Check sheet for the modelled part. Datum: model origin and axes. Units: mm. A direction names the side the tool comes from. Round coordinates to 2 decimals unless told otherwise and drop trailing zeros. Write each loop counter-clockwise with the first axis right and the second up, starting at its lowest first coordinate (ties: lowest second). Pieces come first, ordered by that corner, then holes.
from build123d import *

# Parameters (mm, degrees)
SKETCH1_W           = 91
SKETCH1_H           = 91
SKETCH1_W_2         = 85
SKETCH1_H_2         = 85
BOSS_EXTRUDE1_DEPTH = 40
SKETCH2_W           = 91
SKETCH2_H           = 91
BOSS_EXTRUDE2_DEPTH = 3
FILLET1_R           = 2
SKETCH3_R           = 2.5
BOSS_EXTRUDE3_DEPTH = 3


with BuildPart() as part:
    # Sketch1 → Boss-Extrude1 (new body)
    with BuildSketch(Plane(origin=(0, 0, 0), x_dir=(1, 0, 0), z_dir=(0, 1, 0))):
        with Locations((-42.5, 42.5)):
            Rectangle(SKETCH1_W, SKETCH1_H)
        with Locations((-42.5, 42.5)):
            Rectangle(SKETCH1_W_2, SKETCH1_H_2, mode=Mode.SUBTRACT)
    extrude(amount=BOSS_EXTRUDE1_DEPTH)

    # Sketch2 → Boss-Extrude2 (add)
    with BuildSketch(Plane(origin=(0, 40, 0), x_dir=(1, 0, 0), z_dir=(0, 1, 0))):
        with Locations((-42.5, 42.5)):
            Rectangle(SKETCH2_W, SKETCH2_H)
    extrude(amount=BOSS_EXTRUDE2_DEPTH)

    # Fillet1
    fillet1_edges = [part.edges().sort_by_distance(p)[0] for p in [
        (3, 21.5, -88),
        (3, 21.5, 3),
        (-88, 21.5, 3),
        (-88, 21.5, -88),
    ]]
    fillet(fillet1_edges, radius=FILLET1_R)

    # Sketch3 → Boss-Extrude3 (add)
    with BuildSketch(Plane.XZ.offset(-40)):
        with Locations(Location((-66.5, -29.5, 0), (0, 0, 270))):
            Circle(SKETCH3_R)
        with Locations(Location((-66.5, -55.5, 0), (0, 0, 90))):
            Circle(SKETCH3_R)
        with Locations(Location((-18.5, -55.5, 0), (0, 0, 270))):
            Circle(SKETCH3_R)
        with Locations(Location((-18.5, -29.5, 0), (0, 0, 90))):
            Circle(SKETCH3_R)
    extrude(amount=BOSS_EXTRUDE3_DEPTH)


solid = part.part
1. Sectioned sample at C-C, the plane z = -72.5. Enter the section's corners in (x, y).
2. Sectioned sample at B-B, the plane x = -66.5. Enter the section's corners in (y, z).
3. Sectioned sample at D-D, the plane x = -13. Enter the section's corners in (y, z).
4. Release check for a two-part mould opening along X. For faces 3 (the flat face through (0, 20, -42)), 4 (the flat face through (3, 21, -42)), 5 (the flat face through (-88, 21, -42)) record: released by +X, released by -X, zero draft, split by the parting line, or undercut.
5. Go/stop test with flat-tipped pins: pin 1 (10 mm diameter, centred on x = -35, z = -46.5, fed in from -Y); pin 2 (5.5 mm diameter, centred on x = -19.5, z = -30, fed in from -Y). Record where each tip stops, or that it passes through.
6. Scan lines: line 1 along X through (y, z) = (11.5, -43); line 2 along Y through (x, z) = (-38, -30.5). Record each from-to range of solid material in increasing order.
7. Sectioned sample at A-A, the plane y = 7.5. Enter the section's corners in (x, z).
8. Set-up check for faces 1 (the flat face through (-18, 37, -55)), 2 (the flat face through (-43, 21, 3)): record each of +Z, -Z, +X, -X, +Y, -Y from which the full face is reachable in a straight line by a thin tool's end or side.
Computed values:
1. outline: (-88, 0) - (-85, 0) - (-85, 40) - (0, 40) - (0, 0) - (3, 0) - (3, 43) - (-88, 43) - close
2. outline: (0, -88) - (43, -88) - (43, 3) - (0, 3) - (0, 0) - (40, 0) - (40, -27) - (37, -27) - (37, -32) - (40, -32) - (40, -53) - (37, -53) - (37, -58) - (40, -58) - (40, -85) - (0, -85) - close
3. outline: (0, -88) - (43, -88) - (43, 3) - (0, 3) - (0, 0) - (40, 0) - (40, -85) - (0, -85) - close
4. face 3: undercut
4. face 4: released by +X
4. face 5: released by -X
5. pin 1: stops at y = 40
5. pin 2: stops at y = 37
6. line 1: x = -88 to -85, 0 to 3
6. line 2: y = 40 to 43
7. outline: (-88, -86) arc R2 ccw to (-86, -88) - (1, -88) arc R2 ccw to (3, -86) - (3, 1) arc R2 ccw to (1, 3) - (-86, 3) arc R2 ccw to (-88, 1) - close; hole (-85, -85) - (0, -85) - (0, 0) - (-85, 0) - close
8. face 1: -Y
8. face 2: +Z, +X, -X, +Y, -Y
